Could you check a few things on this model? Use its own coordinates, in mm. A direction names the side the tool comes from. Give positions to 0.01 mm unless a question says otherwise; leave off trailing zeros. Order: outer loops, then holes, each group sorted by start corner. A loop starts at its lowest first (then second) coordinate and runs counter-clockwise, first axis right, second up.
from build123d import *

# Parameters (mm, degrees)
SKETCH10_R           = 7.5
SKETCH10_W           = 20
SKETCH10_H           = 10
SKETCH10_R_2         = 2.6
BOSS_EXTRUDE7_DEPTH  = 3
BOSS_EXTRUDE10_DEPTH = 10
SKETCH12_W           = 3.25
SKETCH12_H           = 56
BOSS_EXTRUDE11_DEPTH = 3
CHAMFER2_SIZE        = 3
CHAMFER3_SIZE        = 3


with BuildPart() as part:
    # Sketch10 → Boss-Extrude7 (new body)
    # profile 1 of 3: a face of its own
    with BuildSketch(Plane.XY):
        Polygon((10, 19.32455532), (10, 31), (-10, 31), (-10, 15.101198027), (-10, -10.060612309), (-10, -31), (10, -31), (10, -17.409211947), align=None)
        with Locations((1, -13)):
            Circle(SKETCH10_R, mode=Mode.SUBTRACT)
        with Locations((1, 13)):
            Circle(SKETCH10_R, mode=Mode.SUBTRACT)
    # profile 2 of 3: a face of its own
    with BuildSketch(Plane.XY):
        with Locations((0, 36)):
            Rectangle(SKETCH10_W, SKETCH10_H)
        with Locations((0, 36)):
            Circle(SKETCH10_R_2, mode=Mode.SUBTRACT)
    # profile 3 of 3: a face of its own
    with BuildSketch(Plane.XY):
        with Locations((0, -36)):
            Rectangle(SKETCH10_W, SKETCH10_H)
        with Locations((0, -36)):
            Circle(SKETCH10_R_2, mode=Mode.SUBTRACT)
    extrude(amount=-BOSS_EXTRUDE7_DEPTH)

    # Sketch9 → Boss-Extrude10 (add)
    with BuildSketch(Plane.XY):
        with BuildLine():
            ThreePointArc((-9.6, 10.026786251), (-1.052303624, 1.988101979), (10, 5.928932188))
            Line((10, 5.928932188), (10, -5.928932188))
            ThreePointArc((10, -5.928932188), (-1.052303624, -1.988101979), (-9.6, -10.026786251))
            Line((-9.6, -10.026786251), (-10, -10.026786251))
            Line((-10, -10.026786251), (-10, 10.026786251))
            Line((-10, 10.026786251), (-9.6, 10.026786251))
        make_face()
        with BuildLine():
            Line((10, 20.071067812), (10, 28))
            Line((10, 28), (-10, 28))
            Line((-10, 28), (-10, 15.973213749))
            Line((-10, 15.973213749), (-9.6, 15.973213749))
            ThreePointArc((-9.6, 15.973213749), (-1.052303624, 24.011898021), (10, 20.071067812))
        make_face()
        with BuildLine():
            Line((-10, -28), (10, -28))
            Line((10, -28), (10, -20.071067812))
            ThreePointArc((10, -20.071067812), (-1.052303624, -24.011898021), (-9.6, -15.973213749))
            Line((-9.6, -15.973213749), (-10, -15.973213749))
            Line((-10, -15.973213749), (-10, -28))
        make_face()
    extrude(amount=-BOSS_EXTRUDE10_DEPTH)

    # Sketch12 → Boss-Extrude11 (add)
    with BuildSketch(Plane(origin=(0, 0, -3), x_dir=(-1, 0, 0), z_dir=(0, 0, -1))):
        with Locations((-11.625, 0)):
            Rectangle(SKETCH12_W, SKETCH12_H)
    extrude(amount=-BOSS_EXTRUDE11_DEPTH)

    # Chamfer2
    chamfer2_edges = [part.edges().sort_by_distance(p)[0] for p in [
        (13.25, -28, -1.5),
    ]]
    chamfer(chamfer2_edges, length=CHAMFER2_SIZE)

    # Chamfer3
    chamfer3_edges = [part.edges().sort_by_distance(p)[0] for p in [
        (13.25, 28, -1.5),
    ]]
    chamfer(chamfer3_edges, length=CHAMFER3_SIZE)


solid = part.part
Item 1: Imagine slicing it at A-A on y = -36. List the corners of the cut face in (x, z) for me.
Findings:
outline: (-10, -3) - (-2.6, -3) - (-2.6, 0) - (-10, 0) - close; (2.6, -3) - (10, -3) - (10, 0) - (2.6, 0) - close
Item 2: For faces 1 (the cylindrical face through (-1.221, 23.975, -6.451)), 2 (the flat face through (10, 34, -1)), 3 (the flat face through (0, -28, -6)), 4 (the flat face through (10, -35, -1)), which set-ups out of +Z, -Z, +X, -X, +Y, -Y let a thin tool reach every point of the face, with its end or its side?
Findings:
face 1: -Z
face 2: +Z, -Z, +X, +Y
face 3: -Z, +X, -X, -Y
face 4: +Z, -Z, +X, -Y
Item 3: Imagine slicing it at B-B on z = -0.75. List the corners of the cut face in (x, y) for me, then the cut area to 3 significant figures.
Findings:
outline: (-10, -41) - (10, -41) - (10, -28) - (10.25, -28) - (13.25, -25) - (13.25, 25) - (10.25, 28) - (10, 28) - (10, 41) - (-10, 41) - close; hole circle Ø15 at (1, -13); hole circle Ø15 at (1, 13); hole circle Ø5.2 at (0, -36); hole circle Ø5.2 at (0, 36)
area: 1,420 mm2
Item 4: Please list where these lines run through material, in increasing order: line 1 along Y through (x, z) = (1, -1.1); line 2 along Y through (x, z) = (0.5, -0.25); line 3 along Y through (x, z) = (7.5, -5).
Findings:
line 1: y = -41 to -38.4, -33.6 to -20.5, -5.5 to 5.5, 20.5 to 33.6, 38.4 to 41
line 2: y = -41 to -38.55, -33.45 to -20.48, -5.52 to 5.52, 20.48 to 33.45, 38.55 to 41
line 3: y = -28 to -22.35, -3.65 to 3.65, 22.35 to 28
Item 5: Imagine slicing it at C-C on z = -8. List the corners of the cut face in (x, y) for me, then the cut area to 3 significant figures.
Findings:
outline: (-10, -28) - (10, -28) - (10, -20.07) arc R11.25 cw to (-9.6, -15.97) - (-10, -15.97) - close; (-10, -10.03) - (-9.6, -10.03) arc R11.25 cw to (10, -5.93) - (10, 5.93) arc R11.25 cw to (-9.6, 10.03) - (-10, 10.03) - close; (-10, 15.97) - (-9.6, 15.97) arc R11.25 cw to (10, 20.07) - (10, 28) - (-10, 28) - close
area: 372 mm2
Item 6: We'd pull the mould along X, two halves only. Please class faces 5 (the cylindrical face through (-1.221, 2.025, -6.451)), 6 (the flat face through (-10, -1, -5)), 7 (the flat face through (2, 1, 0)): +X half, -X half, draft (parallel to the pull), parting line (faces both ways), or undercut.
Findings:
face 5: undercut
face 6: -X half
face 7: draft
Item 7: For pin 1 (2 mm diameter, centred on y = 0, z = -8, fed in from +X); pin 2 (4 mm diameter, centred on x = -4.5, y = -35.5, fed in from -Z); pin 3 (4.5 mm diameter, centred on x = 0, y = -36, fed in from +Z), each with a flat end and sliding along its axis, tell me the tip position at first contact or that it passes through.
Findings:
pin 1: stops at x = 10
pin 2: stops at z = -3
pin 3: passes through
Item 8: Imagine slicing it at D-D on x = 3.75. List the corners of the cut face in (y, z) for me, then the cut area to 3 significant figures.
Findings:
outline: (-41, -3) - (-28, -3) - (-28, -10) - (-23.97, -10) - (-23.97, -3) - (-19.98, -3) - (-19.98, 0) - (-41, 0) - close; (-6.02, -3) - (-2.03, -3) - (-2.03, -10) - (2.03, -10) - (2.03, -3) - (6.02, -3) - (6.02, 0) - (-6.02, 0) - close; (19.98, -3) - (23.97, -3) - (23.97, -10) - (28, -10) - (28, -3) - (41, -3) - (41, 0) - (19.98, 0) - close
area: 247 mm2
